from build123d import *

# Parameters (mm, degrees)
SKETCH1_W           = 54
SKETCH1_H           = 54
BOSS_EXTRUDE1_DEPTH = 5
SKETCH3_W           = 54
SKETCH3_H           = 38
BOSS_EXTRUDE2_DEPTH = 8
SKETCH9_W           = 5.5
SKETCH9_H           = 5
BOSS_EXTRUDE3_DEPTH = 7
SKETCH2_R           = 12
SKETCH2_R_2         = 4.325
SKETCH2_R_3         = 1.85
CUT_EXTRUDE1_DEPTH  = 5
SKETCH4_R           = 2.575
CUT_EXTRUDE2_DEPTH  = 8
SKETCH7_R           = 5.5
CUT_EXTRUDE3_DEPTH  = 4
SKETCH8_W           = 4.486421388
SKETCH8_H           = 2
CUT_EXTRUDE4_DEPTH  = 4
RIB1_REACH          = 72.915
SKETCH5_WALL_W      = 183.428864958
SKETCH5_WALL_H      = 4
RIB9_REACH          = 72.915
SKETCH6_WALL_W      = 183.428864958
SKETCH6_WALL_H      = 6
CHAMFER1_SIZE       = 10
CHAMFER2_SIZE       = 15
CHAMFER3_SIZE       = 15
CHAMFER4_SIZE       = 1
CHAMFER6_SIZE       = 6
LPATTERN2_COUNT     = 2
LPATTERN2_PITCH     = 19.5
CHAMFER7_SIZE       = 2
CHAMFER8_SIZE       = 5


# Some blends are built 0.0001 mm under size
with BuildPart() as part:
    # Sketch1 → Boss-Extrude1 (new body)
    with BuildSketch(Plane(origin=(0, 0, 0), x_dir=(1, 0, 0), z_dir=(0, 1, 0))):
        Rectangle(SKETCH1_W, SKETCH1_H)
    extrude(amount=BOSS_EXTRUDE1_DEPTH)

    # Sketch3 → Boss-Extrude2 (add)
    with BuildSketch(Plane(origin=(0, 0, -27), x_dir=(-1, 0, 0), z_dir=(0, 0, -1))):
        with Locations((0, -14)):
            Rectangle(SKETCH3_W, SKETCH3_H)
    extrude(amount=-BOSS_EXTRUDE2_DEPTH)

    # Sketch9 → Boss-Extrude3 (add)
    with BuildSketch(Plane(origin=(0, 5, 0), x_dir=(1, 0, 0), z_dir=(0, 1, 0))):
        with Locations((10, 29.5)):
            Rectangle(SKETCH9_W, SKETCH9_H)
        with Locations((-10, 29.5)):
            Rectangle(SKETCH9_W, SKETCH9_H)
    boss_extrude3 = extrude(amount=-BOSS_EXTRUDE3_DEPTH)

    # Sketch2 → Cut-Extrude1 (cut)
    with BuildSketch(Plane(origin=(0, 5, 0), x_dir=(1, 0, 0), z_dir=(0, 1, 0))):
        with Locations(Location((-1, -3, 0), (0, 0, 270))):
            Circle(SKETCH2_R)
        with Locations(Location((-18.5, -3, 0), (0, 0, 270))):
            Circle(SKETCH2_R_2)
        with Locations(Location((14.5, 12.5, 0), (0, 0, 270))):
            Circle(SKETCH2_R_3)
        with Locations(Location((-16.5, 12.5, 0), (0, 0, 270))):
            Circle(SKETCH2_R_3)
        with Locations(Location((-16.5, -18.5, 0), (0, 0, 270))):
            Circle(SKETCH2_R_3)
        with Locations(Location((14.5, -18.5, 0), (0, 0, 270))):
            Circle(SKETCH2_R_3)
    extrude(amount=-CUT_EXTRUDE1_DEPTH, mode=Mode.SUBTRACT)

    # Sketch4 → Cut-Extrude2 (cut)
    with BuildSketch(Plane.XY.offset(-19)):
        with Locations((-10, -8)):
            Circle(SKETCH4_R)
        with Locations((10, -8)):
            Circle(SKETCH4_R)
        with Locations((10, -28)):
            Circle(SKETCH4_R)
        with Locations((-10, -28)):
            Circle(SKETCH4_R)
    extrude(amount=-CUT_EXTRUDE2_DEPTH, mode=Mode.SUBTRACT)

    # Sketch7 → Cut-Extrude3 (cut)
    with BuildSketch(Plane.XY.offset(-19)):
        with Locations((-10, -8)):
            Circle(SKETCH7_R)
        with Locations((10, -8)):
            Circle(SKETCH7_R)
        with Locations((10, -28)):
            Circle(SKETCH7_R)
        with Locations((-10, -28)):
            Circle(SKETCH7_R)
    extrude(amount=-CUT_EXTRUDE3_DEPTH, mode=Mode.SUBTRACT)

    # Sketch8 → Cut-Extrude4 (cut)
    with BuildSketch(Plane.XZ):
        with Locations((-13.778117046, 3)):
            Rectangle(SKETCH8_W, SKETCH8_H)
    extrude(amount=-CUT_EXTRUDE4_DEPTH, mode=Mode.SUBTRACT)

    # Sketch5 wall → Rib1 (add, up to next)
    with BuildSketch(Plane(origin=(-27, -14, -5), x_dir=(0, -0.707106781187, -0.707106781187), z_dir=(0, -0.707106781187, 0.707106781187)), mode=Mode.PRIVATE) as rib1_sk1:
        with Locations((0, 2)):
            Rectangle(SKETCH5_WALL_W, SKETCH5_WALL_H)
    rib1_tool1 = extrude(rib1_sk1.sketch, amount=-RIB1_REACH, mode=Mode.PRIVATE) - part.part
    add(rib1_tool1.solids().sort_by_distance((-27, -14, -5))[0])

    # Sketch6 wall → Rib9 (add, up to next)
    with BuildSketch(Plane(origin=(27, -14, -5), x_dir=(0, -0.707106781187, -0.707106781187), z_dir=(0, 0.707106781187, -0.707106781187)), mode=Mode.PRIVATE) as rib9_sk1:
        with Locations((0, 3)):
            Rectangle(SKETCH6_WALL_W, SKETCH6_WALL_H)
    rib9_tool1 = extrude(rib9_sk1.sketch, amount=RIB9_REACH, mode=Mode.PRIVATE) - part.part
    add(rib9_tool1.solids().sort_by_distance((27, -14, -5))[0])

    # Chamfer1
    chamfer1_edges = [part.edges().sort_by_distance(p)[0] for p in [
        (27, 2.5, 27),
        (-27, 2.5, 27),
    ]]
    chamfer(chamfer1_edges, length=CHAMFER1_SIZE)

    # Chamfer2
    # the kernel refuses this chamfer: 15 mm, written as the material it takes off along each edge
    with BuildSketch(Plane(origin=(27, -33, -65.575244819), x_dir=(-0.9996219169112968, -0.02749587661058632, 0), z_dir=(0, 0, 1))) as chamfer2_piece_1:
        Polygon((CHAMFER2_SIZE * 0.999621916911, -CHAMFER2_SIZE * 0.0274958766106), (-CHAMFER2_SIZE * 0.0274958766106, -CHAMFER2_SIZE * 0.999621916911), (0, 0), align=None)
    extrude(amount=85.150489639, mode=Mode.SUBTRACT)

    # Chamfer3
    # the kernel refuses this chamfer: 15 mm, written as the material it takes off along each edge
    with BuildSketch(Plane(origin=(-27, -33, -65.575244819), x_dir=(-0.02749587661058632, 0.9996219169112968, 0), z_dir=(0, 0, 1))) as chamfer3_piece_1:
        Polygon((CHAMFER3_SIZE * 0.999621916911, -CHAMFER3_SIZE * 0.0274958766106), (-CHAMFER3_SIZE * 0.0274958766106, -CHAMFER3_SIZE * 0.999621916911), (0, 0), align=None)
    extrude(amount=85.150489639, mode=Mode.SUBTRACT)

    # Chamfer4
    chamfer4_edges = [part.edges().sort_by_distance(p)[0] for p in [
        (21, -12, -19),
        (-23, -11, -19),
    ]]
    chamfer(chamfer4_edges, length=CHAMFER4_SIZE)

    # Chamfer6
    chamfer6_edges = [part.edges().sort_by_distance(p)[0] for p in [
        (-27, -6.5, -27),
        (27, -6.5, -27),
    ]]
    chamfer(chamfer6_edges, length=CHAMFER6_SIZE)

    # LPattern2: Boss-Extrude3 ×2
    with Locations(*[(0, -i * LPATTERN2_PITCH, 0) for i in range(1, LPATTERN2_COUNT)]):
        add(boss_extrude3)

    # Chamfer7
    chamfer7_edges = [part.edges().sort_by_distance(p)[0] for p in [
        (10, -2, -32),
        (-10, -2, -32),
    ]]
    chamfer(chamfer7_edges, length=CHAMFER7_SIZE)

    # Chamfer8
    chamfer8_edges = [part.edges().sort_by_distance(p)[0] for p in [
        (10, -14.5, -32),
        (-10, -14.5, -32),
    ]]
    chamfer(chamfer8_edges, length=CHAMFER8_SIZE - 0.0001)  # a hair under: the kernel refuses the full size


solid = part.part
Build history of the part. All positions in model axes, mm. A direction names the side the tool comes from. Round coordinates to 2 decimals unless told otherwise and drop trailing zeros. Loops run counter-clockwise (first coordinate to the right, second up) from the corner with the lowest first, then second, coordinate; pieces in that order, holes last. Notation, with made-up numbers: (4.25, 43) -> (21.25, 43) arc R19 ccw to (21.25, 55) -> close; hole circle Ø5 at (43, 59.25). An arc over 180 degrees is marked (long way). One line per item, written item: value. Start each with the question number.
Q1. Two-plate mould, pull along Z, no slides. Class faces 4 (the face through (2.604, 2.535, 14.446)), 5 (the face through (21, -24, -20)), 6 (the face through (22, 2, 22)): released by +Z, released by -Z, zero draft, split by the parting line, or undercut.
Q2. Cut at D-D on z = -17. List the corners of the cut face in (x, y).
Q3. Cut at C-C on z = 3. List the corners of the cut face in (x, y) (3 decimals).
Q4. 3-axis set-ups, long thin cutter, end or side, ignore diameter. For faces 1 (the face through (-7.25, 2, -29)), 2 (the face through (-14, 2, 2)), 3 (the face through (-7.679, -23.014, -20.972)): which of +Z, -Z, +X, -X, +Y, -Y reach the whole face in a straight line?
Q5. Drop flat-ended pins along their axis: pin 1 Ø5 at (x, y) = (-1.5, -29) entering from -Z; pin 2 Ø8 at (y, z) = (-20, -8) entering from +X; pin 3 Ø2.5 at (x, z) = (-11, -28.5) entering from -Y; pin 4 Ø12 at (x, y) = (-7.5, -24) entering from +Z. Give the stop position or say it passes through.
Q6. Cut at B-B on y = -8. List the corners of the cut face in (x, z) (3 decimals).
Q7. Probe line 1 along Y through (x, z) = (-10, -24.85) (3 decimals); line 2 along Y through (x, z) = (-10, -21); line 3 along X through (y, z) = (-28, -20). List the from-to ranges inside material, lowest first.
Q8. Cut at A-A on x = -1. List the corners of the cut face in (y, z).
Computed:
1. face 4: undercut
1. face 5: zero draft
1. face 6: released by +Z
2. outline: (-27, -18) -> (-23, -22) -> (-23, 0) -> (21, 0) -> (21, -24) -> (27, -18) -> (27, 5) -> (-27, 5) -> close
3. outline: (-27, -6) -> (-23, -6) -> (-23, 0) -> (-22.825, 0) -> (-22.825, 5) -> (-27, 5) -> close; (-14.175, 4) -> (-13, 4) -> (-13, 5) -> (-14.175, 5) -> close; (11, 0) -> (21, 0) -> (21, -6) -> (27, -6) -> (27, 5) -> (11, 5) -> close
4. face 1: -Z, +Y, -Y
4. face 2: -Y
4. face 3: +Z
5. pin 1: z = -27
5. pin 2: x = 27
5. pin 3: y = -21.5
5. pin 4: z = -19
6. outline: (-27, -21) -> (-21, -27) -> (-12.575, -27) -> (-12.575, -23) -> (-15.5, -23) -> (-15.5, -19) -> (-22, -19) -> (-23, -18) -> (-23, 1) -> (-27, 1) -> close; (-7.425, -27) -> (7.425, -27) -> (7.425, -23) -> (4.5, -23) -> (4.5, -19) -> (-4.5, -19) -> (-4.5, -23) -> (-7.425, -23) -> close; (12.575, -27) -> (21, -27) -> (27, -21) -> (27, 1) -> (21, 1) -> (21, -18) -> (20, -19) -> (15.5, -19) -> (15.5, -23) -> (12.575, -23) -> close
7. line 1: -33 to -30.575, -25.425 to -10.575, -5.425 to 5
7. line 2: -22.5 to -13.5, -2.5 to 5
7. line 3: -17 to -15.5, -4.5 to 4.5, 15.5 to 17
8. outline: (-33, -27) -> (5, -27) -> (5, -9) -> (0, -9) -> (0, -19) -> (-33, -19) -> close; (0, 15) -> (5, 15) -> (5, 27) -> (0, 27) -> close
